Model file for the job. Use its own axes, mm. Round coordinates to 2 decimals unless told otherwise and drop trailing zeros. Order: outer loops, then holes, each group sorted by start corner. A loop starts at its lowest first (then second) coordinate and runs counter-clockwise, first axis right, second up. Notation, with made-up numbers: (32, 78) - (88, 78) arc R16 ccw to (88, 102) - close; hole circle Ø4 at (63.5, 29). An arc over 180 degrees is marked (long way). Put each result on its own line as item: value. Start each with the question number.
Item 1: Saw through at D-D on z = -12.75. List the corners of the cut face in (x, y).
Item 2: Saw through at B-B on z = -11.25. List the corners of the cut face in (x, y) (3 decimals).
Item 3: Probe probe 1 along Y at (x, z) = (7.75, -11.75). List the from-to ranges inside material, lowest first.
Item 4: Pin check, flat tips, straight feed: pin 1 Ø3 at (x, z) = (5, -4.5) entering from +Y; pin 2 Ø3 at (x, z) = (2.5, -2.5) entering from -Y. Stop position of each tip, or through.
Item 5: Saw through at A-A on x = 3.5. List the corners of the cut face in (y, z) (3 decimals).
Item 6: Saw through at C-C on x = 6. List the corners of the cut face in (y, z).
Autodesk Inventor part; units mm, degrees
ref_plane "YZ Plane" through (0, 0, 0) normal (1, 0, 0) x (0, 1, 0)
ref_plane "XZ Plane" through (0, 0, 0) normal (0, 1, 0) x (-1, 0, 0)
ref_plane "XY Plane" through (0, 0, 0) normal (0, 0, 1) x (1, 0, 0)
sketch "Sketch1" plane through (0, 0, 0) normal (0, 1, 0) x (-1, 0, 0)
  line L0 (0, 0) -> (-10, 0)
  line L1 (-10, 0) -> (-10, -15)
  line L2 (-10, -15) -> (0, -15)
  line L3 (0, -15) -> (0, 0)
  dimension "d0" = 15
  dimension "d1" = 10
extrude "Extrusion1" add sketch "Sketch1" along normal blind 0.23
sketch "Sketch2" plane through (0, 0.23, 0) normal (0, 1, 0) x (1, 0, 0)
  line L0 (4.68, 10.01) -> (3.2, 10.01)
  line L1 (3.2, 10.01) -> (3.2, 11.99)
  line L2 (3.2, 11.99) -> (4.68, 11.99)
  line L3 (4.68, 11.99) -> (4.68, 10.01)
  line L4 (1.48, 10.01) -> (0, 10.01)
  line L5 (0, 10.01) -> (0, 11.99)
  line L6 (0, 11.99) -> (1.48, 11.99)
  line L7 (1.48, 11.99) -> (1.48, 10.01)
  line L8 (0, 11.99) -> (1.48, 10.01) construction
  line L9 (3.2, 11.99) -> (4.68, 10.01) construction
  line L10 (10, 15) -> (0, 15) construction
  line L11 (10, 0) -> (10, 15) construction
  line L12 (0, 15) -> (0, 0)
  point P0 (0.74, 11)
  point P1 (3.94, 11)
  dimension "d4" = 3.2
  dimension "d5" = 4
  dimension "d6" = 1.48
  dimension "d7" = 1.98
extrude "Extrusion2" add sketch "Sketch2" along normal blind 0.035
properties part number "Antenna" material "Copper, Wrought"
Results found:
1. outline: (0, 0) - (10, 0) - (10, 0.23) - (0, 0.23) - close
2. outline: (0, 0) - (10, 0) - (10, 0.23) - (4.68, 0.23) - (4.68, 0.265) - (3.2, 0.265) - (3.2, 0.23) - (1.48, 0.23) - (1.48, 0.265) - (0, 0.265) - close
3. probe 1: y = 0 to 0.23
4. pin 1: stops at y = 0.23
4. pin 2: stops at y = 0
5. outline: (0, -15) - (0.23, -15) - (0.23, -11.99) - (0.265, -11.99) - (0.265, -10.01) - (0.23, -10.01) - (0.23, 0) - (0, 0) - close
6. outline: (0, -15) - (0.23, -15) - (0.23, 0) - (0, 0) - close
